```python
from build123d import *

# Parameters (mm, degrees)
BASE_FLANGE1_DEPTH             = 1.5
EDGE_FLANGE1_STRIP_W           = 6.4
EDGE_FLANGE1_STRIP_H           = 1.5
EDGE_FLANGE1_STRIP_CUT_DEPTH   = 151.65
EDGE_FLANGE1_STRIP_2_W         = 6.4
EDGE_FLANGE1_STRIP_2_H         = 1.5
EDGE_FLANGE1_STRIP_CUT_2_DEPTH = 196.65
EDGE_FLANGE1_DEPTH             = 151.65
EDGE_FLANGE1_BEND_DEPTH        = 196.65


# Sheet-metal steps are written as plain solids
with BuildPart() as part:
    # Sketch1 → Base-Flange1 (new body)
    with BuildSketch(Plane.XY):
        with BuildLine():
            Line((13.35, 0), (13.35, 13.35))
            Line((13.35, 13.35), (210, 13.35))
            Line((210, 13.35), (210, -1.65))
            Line((210, -1.65), (50, -31.65))
            Line((50, -31.65), (-50, -31.65))
            Line((-50, -31.65), (-165, -1.65))
            Line((-165, -1.65), (-165, 13.35))
            Line((-165, 13.35), (-13.35, 13.35))
            Line((-13.35, 13.35), (-13.35, 0))
            ThreePointArc((-13.35, 0), (0, -13.35), (13.35, 0))
        make_face()
    extrude(amount=-BASE_FLANGE1_DEPTH)

    # Edge-Flange1 strip (across the edge) → Edge-Flange1 strip cut (cut)
    with BuildSketch(Plane(origin=(-13.35, 13.35, 0), x_dir=(0, -1, 0), z_dir=(-1, 0, 0))):
        with Locations((-1.5, -0.75)):
            Rectangle(EDGE_FLANGE1_STRIP_W, EDGE_FLANGE1_STRIP_H)
    extrude(amount=EDGE_FLANGE1_STRIP_CUT_DEPTH, mode=Mode.SUBTRACT)

    # Edge-Flange1 strip 2 (across the edge) → Edge-Flange1 strip cut 2 (cut)
    with BuildSketch(Plane(origin=(210, 13.35, 0), x_dir=(0, -1, 0), z_dir=(-1, 0, 0))):
        with Locations((-1.5, -0.75)):
            Rectangle(EDGE_FLANGE1_STRIP_2_W, EDGE_FLANGE1_STRIP_2_H)
    extrude(amount=EDGE_FLANGE1_STRIP_CUT_2_DEPTH, mode=Mode.SUBTRACT)

    # Edge-Flange1 section (across the edge) → Edge-Flange1 (add)
    with BuildSketch(Plane(origin=(-13.35, 13.35, 0), x_dir=(0, -1, 0), z_dir=(-1, 0, 0))):
        with BuildLine():
            Line((0, 0.2), (0, 18.5))
            Line((0, 18.5), (1.5, 18.5))
            Line((1.5, 18.5), (1.5, 0.2))
            ThreePointArc((1.5, 0.2), (1.558578644, 0.058578644), (1.7, 0))
            Line((1.7, 0), (1.7, -1.5))
            ThreePointArc((1.7, -1.5), (0.497918472, -1.002081528), (0, 0.2))
        make_face()
    extrude(amount=EDGE_FLANGE1_DEPTH)

    # Edge-Flange1 section 2 (across the edge) → Edge-Flange1 bend (add)
    with BuildSketch(Plane(origin=(210, 13.35, 0), x_dir=(0, -1, 0), z_dir=(-1, 0, 0))):
        with BuildLine():
            Line((0, 0.2), (0, 18.5))
            Line((0, 18.5), (1.5, 18.5))
            Line((1.5, 18.5), (1.5, 0.2))
            ThreePointArc((1.5, 0.2), (1.558578644, 0.058578644), (1.7, 0))
            Line((1.7, 0), (1.7, -1.5))
            ThreePointArc((1.7, -1.5), (0.497918472, -1.002081528), (0, 0.2))
        make_face()
    extrude(amount=EDGE_FLANGE1_BEND_DEPTH)


solid = part.part
```
Input: part model. Units: mm. Frame: model coordinates. A direction names the side the tool comes from. Give positions to 0.01 mm unless a question says otherwise; leave off trailing zeros. Order: outer loops, then holes, each group sorted by start corner. A loop starts at its lowest first (then second) coordinate and runs counter-clockwise, first axis right, second up. Notation, with made-up numbers: M -0.75,89.25 L 45.25,89.25 A32 ccw 45.25,115.25 Z; hole C 4,-12 d9. An arc over 180 degrees is marked long. One line per question, with ' | ' between items.
1) Section D-D on y = -23.5. Output: boundary loops of the cut face in (x, z), and give its area (3 significant figures).
Filled in:
outline: M -81.24,-1.5 L 93.47,-1.5 L 93.47,0 L -81.24,0 Z | area: 262 mm2
2) Section B-B on y = 5.5. Output: boundary loops of the cut face in (x, z).
Filled in:
outline: M -165,-1.5 L -13.35,-1.5 L -13.35,0 L -165,0 Z; M 13.35,-1.5 L 210,-1.5 L 210,0 L 13.35,0 Z
3) Ray query, L1, parallel to Z at x = -30.5, y = 11; L2, parallel to Y at x = -28.5, z = 1.25. Return the intervals inside material, ascending.
Filled in:
L1: z = -1.5 to 0 | L2: y = 11.85 to 13.35
4) Access query for faces 5 (the face through (-106.7, -16.86, -0.74)), 6 (the face through (13.35, 12, 6)), 7 (the face through (25, -5, 0)). Directions: +Z, -Z, +X, -X, +Y, -Y. A direction counts if a zero-diameter tool reaches every point of the face in a straight line with its end or side. Return the directions, or none.
Filled in:
face 5: +Z, -Z, -X, -Y | face 6: +Z, -Z, +Y | face 7: +Z, +X, -X, -Y
5) Section C-C on x = 54.5. Output: boundary loops of the cut face in (y, z), and give its area (3 significant figures).
Filled in:
outline: M -30.81,-1.5 L 11.65,-1.5 A1.7 ccw 13.35,0.2 L 13.35,18.5 L 11.85,18.5 L 11.85,0.2 A0.2 cw 11.65,0 L -30.81,0 Z | area: 93.4 mm2
6) Draft query along X for faces 1 (the face through (-0.294, -13.347, -0.74)), 2 (the face through (210, 12, 6)), 3 (the face through (25, -5, -1.5)), 4 (the face through (-13.35, 12, 6)). Return one class per face: pulls with the +X half, pulls with the -X half, needs draft (parallel to the pull), parting line crosses it, or undercut.
Filled in:
face 1: undercut | face 2: pulls with the +X half | face 3: needs draft | face 4: undercut
7) Section A-A on z = 4.25. Output: boundary loops of the cut face in (x, y), and give its area (3 significant figures).
Filled in:
outline: M -165,11.85 L -13.35,11.85 L -13.35,13.35 L -165,13.35 Z; M 13.35,11.85 L 210,11.85 L 210,13.35 L 13.35,13.35 Z | area: 522 mm2
8) Contact query for flat-ended pins moving along their axis: P1, Ø5.5, axis at x = -79, z = 11.5, coming from the -Y side; P2, Ø10, axis at y = 6.5, z = 4, coming from the -X side; P3, Ø12, axis at x = 65.5, y = -14.5, coming from the +Z side. Output: stop coordinate, or through.
Filled in:
P1: stops at y = 11.85 | P2: stops at x = -165 | P3: stops at z = 0
